from build123d import *

# Parameters (mm, degrees)
F0_R     = 2
F0_R_2   = 1.5
F1_DEPTH = 8
F3_DEPTH = 2.5
F5_DEPTH = 2.5
F7_DEPTH = 2.5
F9_DEPTH = 3.1


with BuildPart() as f1:
    # F0 (on Top) → F1 (new body)
    with BuildSketch(Plane.XY):
        with BuildLine():
            ThreePointArc((3, 42.922839), (5.91608, 45.505737), (7, 49.247394))
            ThreePointArc((7, 49.247394), (0, 56.247394), (-7, 49.247394))
            ThreePointArc((-7, 49.247394), (-3.741657, 43.331314), (3, 42.922839))
        make_face()
        with Locations((0, 49.247394)):
            Circle(F0_R, mode=Mode.SUBTRACT)
        with BuildLine():
            ThreePointArc((3, 42.922839), (-3.741657, 43.331314), (-7, 49.247394))
            Line((-7, 49.247394), (-7, 14.247394))
            Line((-7, 14.247394), (-6.985994, 13.804799))
            Line((-6.985994, 13.804799), (-4.5, -64.752606))
            ThreePointArc((-4.5, -64.752606), (0, -69.252606), (4.5, -64.752606))
            Line((4.5, -64.752606), (6.996488, 14.025675))
            ThreePointArc((6.996488, 14.025675), (5.974602, 17.894877), (3, 20.571949))
            Line((3, 20.571949), (3, 42.922839))
        make_face()
        with Locations((0, -64.752606)):
            Circle(F0_R_2, mode=Mode.SUBTRACT)
        with Locations((0, 14.247394)):
            Circle(F0_R, mode=Mode.SUBTRACT)
        with BuildLine():
            Line((-6.985994, 13.804799), (-7, 14.247394))
            ThreePointArc((-7, 14.247394), (-6.996498, 14.025986), (-6.985994, 13.804799))
        make_face()
    extrude(amount=F1_DEPTH)

    # F2 (on face) → F3 (cut)
    with BuildSketch(Plane.XY.offset(8)):
        with BuildLine():
            Line((4, 2.52692), (3.994938, 2.325746))
            ThreePointArc((3.994938, 2.325746), (3.998734, 2.426301), (4, 2.52692))
        make_face()
        with BuildLine():
            Line((2.499209, -57.116628), (3.994938, 2.325746))
            Line((3.994938, 2.325746), (4, 2.52692))
            ThreePointArc((4, 2.52692), (0, 6.52692), (-4, 2.52692))
            Line((-4, 2.52692), (-3.994938, 2.325746))
            Line((-3.994938, 2.325746), (-2.499209, -57.116628))
            ThreePointArc((-2.499209, -57.116628), (0, -59.553741), (2.499209, -57.116628))
        make_face()
        with BuildLine():
            Line((-3.994938, 2.325746), (-4, 2.52692))
            ThreePointArc((-4, 2.52692), (-3.998734, 2.426301), (-3.994938, 2.325746))
        make_face()
    extrude(amount=-F3_DEPTH, mode=Mode.SUBTRACT)

    # F4 (on face) → F5 (cut)
    with BuildSketch(Plane.XY.offset(8)):
        with BuildLine():
            Line((0, 23.537273), (0, 39.860327))
            ThreePointArc((0, 39.860327), (-2, 41.860327), (-4, 39.860327))
            Line((-4, 39.860327), (-4, 23.537273))
            ThreePointArc((-4, 23.537273), (-2, 21.537273), (0, 23.537273))
        make_face()
    extrude(amount=-F5_DEPTH, mode=Mode.SUBTRACT)

    # F6 (on face) → F7 (cut)
    with BuildSketch(Plane(origin=(0, 0, 0), x_dir=(1, 0, 0), z_dir=(0, 0, -1))):
        with BuildLine():
            Line((-4.5, -24.484327), (-4.5, -39.479643))
            ThreePointArc((-4.5, -39.479643), (-2, -41.979643), (0.5, -39.479643))
            Line((0.5, -39.479643), (0.5, -24.484327))
            ThreePointArc((0.5, -24.484327), (-2, -21.984327), (-4.5, -24.484327))
        make_face()
    extrude(amount=-F7_DEPTH, mode=Mode.SUBTRACT)

    # F8 (on face) → F9 (cut)
    with BuildSketch(Plane(origin=(0, 0, 0), x_dir=(1, 0, 0), z_dir=(0, 0, -1))):
        with BuildLine():
            Line((-4.5, -2.380997), (-4.48963, -2.075676))
            ThreePointArc((-4.48963, -2.075676), (-4.497407, -2.228248), (-4.5, -2.380997))
        make_face()
        with BuildLine():
            Line((-2.498559, 56.54796), (-4.48963, -2.075676))
            Line((-4.48963, -2.075676), (-4.5, -2.380997))
            ThreePointArc((-4.5, -2.380997), (0, -6.880997), (4.5, -2.380997))
            Line((4.5, -2.380997), (4.48963, -2.075676))
            Line((4.48963, -2.075676), (2.498559, 56.54796))
            ThreePointArc((2.498559, 56.54796), (0, 58.9631), (-2.498559, 56.54796))
        make_face()
        with BuildLine():
            Line((4.48963, -2.075676), (4.5, -2.380997))
            ThreePointArc((4.5, -2.380997), (4.497407, -2.228248), (4.48963, -2.075676))
        make_face()
    extrude(amount=-F9_DEPTH, mode=Mode.SUBTRACT)


solid = f1.part
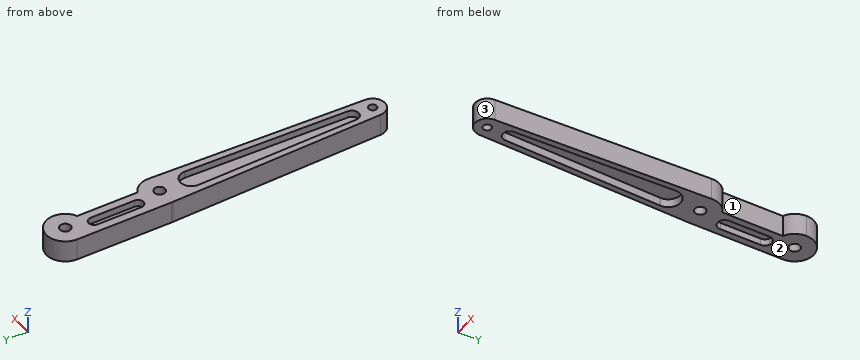
Geometry: final body of the model. Coordinates: model frame, mm. Face numbers are marked on the shaded views. Coordinates: 2 decimals unless noted, no trailing zeros. Loops run counter-clockwise (first coordinate to the right, second up) from the corner with the lowest first, then second, coordinate; pieces in that order, holes last. Notation, with made-up numbers: M -30,4 L -12,4 A23 ccw -12,37 Z; hole C 84.5,14.25 d9. An arc over 180 degrees is marked long. One line per item, written item: value. Start each with the question number.
1) Cut plane A-A (x = 5.75). Return loops of the section in (y, z).
2) Pin query (flat end, axial travel): P1, Ø2.5, axis at x = 0, y = -64.75, coming from the +Z side; P2, Ø3, axis at y = 31.5, z = 1, coming from the +X side; P3, Ø2.5, axis at x = 1, y = -30, coming from the -Z side; P4, Ø3, axis at y = -28, z = 4.5, coming from the +X side. Return the tip coordinate at first contact, or that it passes through.
3) Cut plane B-B (y = -30.5). Return loops of the section in (x, z), then the cut area to 3 significant figures.
4) Material intervals for L1, parallel to X at y = 14, z = 7.25; L2, parallel to X at y = 35, z = 7; L3, parallel to Y at x = 0, z = 2.25, sorted ascending. Write a range as from..to.
5) Draft query along Y for the marked faces 1, 2 and 3. Return one class per face: released by +Y, released by -Y, zero draft, split by the parting line, or undercut.
6) Cut plane C-C (y = 26). Return loops of the section in (x, z), then the cut area to 3 significant figures.
Evaluation:
1. outline: M -25.31,0 L 18.24,0 L 18.24,8 L -25.31,8 Z; M 45.26,0 L 53.24,0 L 53.24,8 L 45.26,8 Z
2. P1: through
2. P2: x = 3
2. P3: z = 3.1
2. P4: x = 5.71
3. outline: M -5.58,0 L -3.38,0 L -3.38,3.1 L 3.38,3.1 L 3.38,0 L 5.59,0 L 5.59,8 L 3.17,8 L 3.17,5.5 L -3.17,5.5 L -3.17,8 L -5.58,8 Z
3. area: 52.5 mm^2
4. L1: -7..-1.98, 1.98..7
4. L2: -7..-4, 0..3
4. L3: -69.25..-66.25, -63.25..-58.96, 6.88..12.25, 16.25..22.98, 40.98..47.25, 51.25..56.25
5. face 1: undercut
5. face 2: zero draft
5. face 3: released by -Y
6. outline: M -7,0 L -4.5,0 L -4.5,2.5 L 0.5,2.5 L 0.5,0 L 3,0 L 3,8 L 0,8 L 0,5.5 L -4,5.5 L -4,8 L -7,8 Z
6. area: 57.5 mm^2
